Verification items for the finished model (mm, model axes). Give positions to 0.01 mm unless a question says otherwise; leave off trailing zeros. Loops run counter-clockwise (first coordinate to the right, second up) from the corner with the lowest first, then second, coordinate; pieces in that order, holes last. Notation, with made-up numbers: (-35.75, -6.5) - (22.25, -6.5) arc R14 cw to (22.25, 11.5) - close; hole circle Ø6 at (69.5, 5). An arc over 180 degrees is marked (long way). Use one line per item in the form item = value.
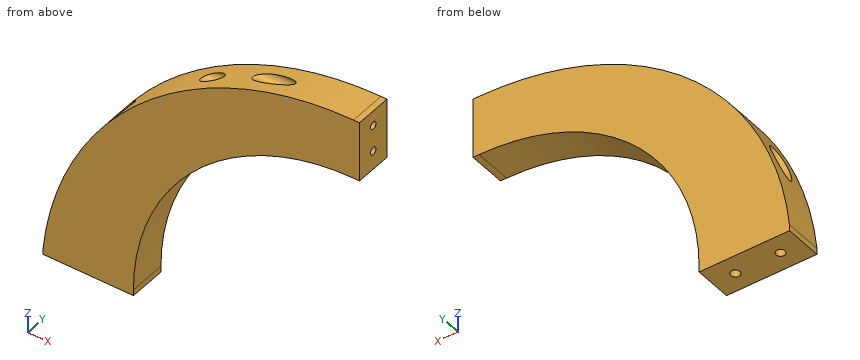
```python
from build123d import *

# Parameters (mm, degrees)
F1_DEPTH      = 12.5
F2_R          = 2.5
F3_DEPTH      = 4
F4_R          = 4.5
F5_DEPTH      = 206.001
F6_R          = 3
F7_DEPTH      = 5
F8_R          = 6
F9_DEPTH      = 185.0010001
F10_S5_R      = 3
F10_T6_DEPTH  = 10
F10_S11_R     = 3
F10_T12_DEPTH = 10


# Not quite as in the source:
# - a fillet or chamfer that OpenCascade refuses, or shapes differently, is made with other operations: its cross-section is extruded or revolved along the edge and cut away or added


with BuildPart() as f1:
    # F0 (on Front) → F1 (new body, symmetric)
    with BuildSketch(Plane.XZ):
        with BuildLine():
            Line((0, 150), (0, 190))
            Line((0, 190), (-4, 190))
            ThreePointArc((-4, 190), (-142.7731962592, 136.6197765021), (-210, 4))
            Line((-210, 4), (-210, 0))
            Line((-210, 0), (-150, 0))
            Line((-150, 0), (-150, 4))
            ThreePointArc((-150, 4), (-107.2375900532, 107.2375900532), (-4, 150))
            Line((-4, 150), (0, 150))
        make_face()
    extrude(amount=F1_DEPTH, both=True)

    # F2 (on face) → F3 (cut)
    with BuildSketch(Plane.YZ):
        with Locations((0, 180)):
            Circle(F2_R)
        with Locations((0, 162.5)):
            Circle(F2_R)
    extrude(amount=-F3_DEPTH, mode=Mode.SUBTRACT)

    # F4 (on face) → F5 (cut, through all)
    with BuildSketch(Plane.YZ.offset(-4)):
        with Locations((0, 180)):
            Circle(F4_R)
        with Locations((0, 162.5)):
            Circle(F4_R)
    extrude(amount=-F5_DEPTH, mode=Mode.SUBTRACT)

    # F6 (on face) → F7 (cut)
    with BuildSketch(Plane(origin=(0, 0, 0), x_dir=(1, 0, 0), z_dir=(0, 0, -1))):
        with Locations((-165, 0)):
            Circle(F6_R)
        with Locations((-195, 0)):
            Circle(F6_R)
    extrude(amount=-F7_DEPTH, mode=Mode.SUBTRACT)

    # F8 (on face) → F9 (cut, through all)
    with BuildSketch(Plane(origin=(0, 0, 5), x_dir=(1, 0, 0), z_dir=(0, 0, -1))):
        with Locations((-165, 0)):
            Circle(F8_R)
        with Locations((-195, 0)):
            Circle(F8_R)
    extrude(amount=-F9_DEPTH, mode=Mode.SUBTRACT)

    # F10: chamfer of 5 on 2 edges, made by hand


with BuildPart() as f10_tool2:
    # F10_s3 → F10_t4 (revolve)
    with BuildSketch(Plane.XZ):
        Polygon((-189, 10), (-194, 5), (-189, 5), align=None)
    revolve(axis=Axis((-195, 0, 5), (0, 0, -1)))

    # F10_s5 → F10_t6 (cut, symmetric)
    with BuildSketch(Plane.XY.offset(7.5)):
        with Locations((-195, 0)):
            Circle(F10_S5_R)
    extrude(amount=F10_T6_DEPTH, both=True, mode=Mode.SUBTRACT)


with BuildPart() as f1_1:
    add(f1.part)

    # F10_t1: union F10_tool2
    add(f10_tool2.part)


with BuildPart() as f10_tool8:
    # F10_s9 → F10_t10 (revolve)
    with BuildSketch(Plane.XZ):
        Polygon((-159, 10), (-164, 5), (-159, 5), align=None)
    revolve(axis=Axis((-165, 0, 5), (0, 0, -1)))

    # F10_s11 → F10_t12 (cut, symmetric)
    with BuildSketch(Plane.XY.offset(7.5)):
        with Locations((-165, 0)):
            Circle(F10_S11_R)
    extrude(amount=F10_T12_DEPTH, both=True, mode=Mode.SUBTRACT)


with BuildPart() as f1_2:
    add(f1_1.part)

    # F10_t7: union F10_tool8
    add(f10_tool8.part)


solid = f1_2.part
```
1. Section check D-D, the plane y = 0. State how many separate pieces and enclosed holes the cut face has, then the cut area to 3 significant figures.
Result set:
separate_pieces = 5
enclosed_holes = 0
area = 9,440 mm²
2. Scan lines: probe 1 along Z at (x, y) = (-2.85, 0); probe 2 along Y at (x, z) = (-195, 3.5); probe 3 along X at (y, z) = (0, 44). Record each from-to range of solid material in increasing order.
Result set:
probe_1 = 150 to 160, 165 to 177.5, 182.5 to 190
probe_2 = -12.5 to -3, 3 to 12.5
probe_3 = -201.86 to -201, -189 to -171, -159 to -144.41
3. Depth check by flat-ended pin: pin 1 Ø5 at (x, y) = (-156, 9.5) entering from +Z; pin 2 Ø2 at (x, y) = (-159, -4.5) entering from +Z; pin 3 Ø1 at (x, y) = (-98.5, -9) entering from -Z. Enter the tip coordinate at first touch or a pass-through.
Result set:
pin_1 = 126.21
pin_2 = 121.36
pin_3 = 114.86
4. Section check C-C, the plane z = 86. Record the cut outline in (x, y).
Result set:
outline = (-183.6, -12.5) - (-124.8, -12.5) - (-124.8, 12.5) - (-183.6, 12.5) - close; hole circle Ø12 at (-165, 0)
5. Section check A-A, the plane x = -195. Record the cut outline in (y, z), then the cut area to 3 significant figures.
Result set:
outline = (-12.5, 0) - (-3, 0) - (-3, 7) - (-6, 10) - (-6, 62.92) - (-12.5, 62.92) - close; (3, 0) - (12.5, 0) - (12.5, 62.92) - (6, 62.92) - (6, 10) - (3, 7) - close
area = 869 mm²
6. Section check B-B, the plane z = 180. Record the cut outline in (x, y), then the cut area to 3 significant figures.
Result set:
outline = (-67.57, -12.5) - (0, -12.5) - (0, -2.5) - (-4, -2.5) - (-4, -4.5) - (-67.57, -4.5) - close; (-67.57, 4.5) - (-4, 4.5) - (-4, 2.5) - (0, 2.5) - (0, 12.5) - (-67.57, 12.5) - close
area = 1,100 mm²
